```python
from build123d import *

# Parameters (mm, degrees)
AUFSATZ_LINEAR_AUSTRAGEN1_DEPTH      = 40
AUFSATZ_LINEAR_AUSTRAGEN2_DEPTH      = 10
SCHNITT_LINEAR_AUSTRAGEN1_DEPTH      = 20
SKIZZE5_R                            = 1.75
SCHNITT_LINEAR_AUSTRAGEN2_DEPTH      = 1
SCHNITT_LINEAR_AUSTRAGEN2_DEPTH_BACK = 21


with BuildPart() as part:
    # Skizze1 → Aufsatz-Linear austragen1 (new body)
    with BuildSketch(Plane.XY):
        Polygon((0, 5), (0, -5), (4, -5), (4, -10), (11, -10), (11, 10), (4, 10), (4, 5), align=None)
    extrude(amount=AUFSATZ_LINEAR_AUSTRAGEN1_DEPTH)

    # Skizze2 → Aufsatz-Linear austragen2 (add)
    with BuildSketch(Plane(origin=(0, 5, 0), x_dir=(1, 0, 0), z_dir=(0, 1, 0))):
        Polygon((0, -40), (-12.044350914, -8.623393141), (0, -4), align=None)
    extrude(amount=-AUFSATZ_LINEAR_AUSTRAGEN2_DEPTH)

    # Skizze4 → Schnitt-Linear austragen1 (cut)
    with BuildSketch(Plane(origin=(0, 10, 0), x_dir=(1, 0, 0), z_dir=(0, 1, 0))):
        Polygon((-10.985237261, -8.216837501), (0, -8.216837501), (11, -15), (11, 0), (0, 0), (0, -4), align=None)
    extrude(amount=-SCHNITT_LINEAR_AUSTRAGEN1_DEPTH, mode=Mode.SUBTRACT)

    # Skizze5 → Schnitt-Linear austragen2 (cut, two sides)
    with BuildSketch(Plane(origin=(0, 10, 0), x_dir=(1, 0, 0), z_dir=(0, 1, 0))) as schnitt_linear_austragen2_sk:
        with Locations((0, -25)):
            Circle(SKIZZE5_R)
        with Locations((0, -11.5)):
            Circle(SKIZZE5_R)
    extrude(amount=SCHNITT_LINEAR_AUSTRAGEN2_DEPTH, mode=Mode.SUBTRACT)
    extrude(schnitt_linear_austragen2_sk.sketch, amount=-SCHNITT_LINEAR_AUSTRAGEN2_DEPTH_BACK, mode=Mode.SUBTRACT)


solid = part.part
```
For this review, take the finished solid that the model builds, in its own axes (mm). A direction names the side the tool comes from. Round coordinates to 2 decimals unless told otherwise and drop trailing zeros. Loops run counter-clockwise (first coordinate to the right, second up) from the corner with the lowest first, then second, coordinate; pieces in that order, holes last.
Q1. Add section A-A on z = 11.5. Write out the cut boundary in (x, y).
Result sheet:
outline: (-10.94, -5) - (-1.75, -5) - (-1.75, 5) - (-10.94, 5) - close; (1.75, -5) - (4, -5) - (4, -10) - (5.32, -10) - (5.32, 10) - (4, 10) - (4, 5) - (1.75, 5) - close
Q2. Add section C-C on y = -5.75. Write out the cut boundary in (x, z), plus the area to 3 significant figures.
Result sheet:
outline: (4, 10.68) - (11, 15) - (11, 40) - (4, 40) - close
area: 190 mm2
Q3. Add section D-D on z = 25. Write out the cut boundary in (x, y), plus the area to 3 significant figures.
Result sheet:
outline: (-5.76, -5) - (-1.75, -5) - (-1.75, 5) - (-5.76, 5) - close; (1.75, -5) - (4, -5) - (4, -10) - (11, -10) - (11, 10) - (4, 10) - (4, 5) - (1.75, 5) - close
area: 203 mm2
Q4. Insertion check: pin 1 Ø8 at (x, z) = (-5, 19) entering from +Y; pin 2 Ø5.5 at (y, z) = (6.5, 29) entering from -X; pin 3 Ø5 at (x, z) = (-1.5, 29.5) entering from -Y; pin 4 Ø10 at (x, y) = (-1, -1) entering from +Z. Each pin has a flat end and moves straight along its axis. Give the tip position at first contact, or say it passes through.
Result sheet:
pin 1: stops at y = 5
pin 2: stops at x = -5.11
pin 3: stops at y = -5
pin 4: stops at z = 40
Q5. Machinability: for faces 1 (the face through (-2, 5, 20)), 2 (the face through (7, -10, 25)), 3 (the face through (-2, -5, 20)), which of the approach directions +Z, -Z, +X, -X, +Y, -Y give a long, thin tool a straight path to every point of the face, cutting with its end or side? Answer none if there is none.
Result sheet:
face 1: +Z, -Z, -X, +Y
face 2: +Z, -Z, +X, -X, -Y
face 3: +Z, -Z, -X, -Y
Q6. Add section B-B on y = -1.75. Write out the cut boundary in (x, z).
Result sheet:
outline: (-12.04, 8.62) - (-10.99, 8.22) - (0, 8.22) - (11, 15) - (11, 40) - (0, 40) - close; hole circle Ø3.5 at (0, 11.5); hole circle Ø3.5 at (0, 25)
Q7. To check wall thickness, follow line 1 along Y through (x, z) = (-7.5, 17.5); line 2 along X through (y, z) = (-8.5, 23); line 3 along X through (y, z) = (0.5, 11.5). State the ranges of each line that lie inside material, in increasing order.
Result sheet:
line 1: y = -5 to 5
line 2: x = 4 to 11
line 3: x = -10.94 to -1.75, 1.75 to 5.32
Q8. Mouldability with a two-part tool opening along Z and no side actions: class faces 4 (the face through (8, 10, 25)), 5 (the face through (-0.228, 0.07, 23.265)), 6 (the face through (-0.228, 0.07, 9.765)), 7 (the face through (-5.94, 0.07, 24.53)) as +Z half, -Z half, draft (parallel to the pull), parting line (faces both ways), or undercut.
Result sheet:
face 4: draft
face 5: undercut
face 6: undercut
face 7: +Z half
